```python
from build123d import *

# Parameters (mm, degrees)
SKETCH2_W           = 34
SKETCH2_H           = 34
BOSS_EXTRUDE2_DEPTH = 35
CUT_EXTRUDE6_DEPTH  = 35
SKETCH17_W          = 30
SKETCH17_H          = 30
CUT_EXTRUDE7_DEPTH  = 10
SKETCH18_W          = 30
SKETCH18_H          = 10
CUT_EXTRUDE8_DEPTH  = 30
SKETCH19_R          = 11
CUT_EXTRUDE10_DEPTH = 7
SKETCH20_R          = 11
CUT_EXTRUDE11_DEPTH = 7
SKETCH22_R          = 4
CUT_EXTRUDE12_DEPTH = 30


with BuildPart() as part:
    # Sketch2 → Boss-Extrude2 (new body)
    with BuildSketch(Plane(origin=(0, 0, 0), x_dir=(1, 0, 0), z_dir=(0, 1, 0))):
        Rectangle(SKETCH2_W, SKETCH2_H)
    boss_extrude2 = extrude(amount=BOSS_EXTRUDE2_DEPTH)

    # Sketch16 → Cut-Extrude6 (cut)
    with BuildSketch(Plane.XY.offset(17)):
        Polygon((-17, 35), (-17, 10.991783965), (17, 35), align=None)
    extrude(amount=-CUT_EXTRUDE6_DEPTH, mode=Mode.SUBTRACT)

    # Sketch17 → Cut-Extrude7 (cut)
    with BuildSketch(Plane.XZ):
        Rectangle(SKETCH17_W, SKETCH17_H)
    cut_extrude7 = extrude(amount=-CUT_EXTRUDE7_DEPTH, mode=Mode.SUBTRACT)

    # Mirror6: Boss-Extrude2, Cut-Extrude7 across plane
    add(boss_extrude2.mirror(Plane(origin=(17, 35, -18), x_dir=(0, 0, 1), z_dir=(0.57681494, -0.816874853, 0))))
    add(cut_extrude7.mirror(Plane(origin=(17, 35, -18), x_dir=(0, 0, 1), z_dir=(0.57681494, -0.816874853, 0))), mode=Mode.SUBTRACT)

    # Sketch18 → Cut-Extrude8 (cut)
    with BuildSketch(Plane.ZY.offset(-15)):
        with Locations((0, 5)):
            Rectangle(SKETCH18_W, SKETCH18_H)
    extrude(amount=CUT_EXTRUDE8_DEPTH, mode=Mode.SUBTRACT)

    # Sketch19 → Cut-Extrude10 (cut)
    with BuildSketch(Plane(origin=(0, 0, -17), x_dir=(-1, 0, 0), z_dir=(0, 0, -1))):
        with Locations((0, 22.995891982)):
            Circle(SKETCH19_R)
    extrude(amount=-CUT_EXTRUDE10_DEPTH, mode=Mode.SUBTRACT)

    # Sketch20 → Cut-Extrude11 (cut)
    with BuildSketch(Plane.XY.offset(17)):
        with Locations((0, 22.995891982)):
            Circle(SKETCH20_R)
    extrude(amount=-CUT_EXTRUDE11_DEPTH, mode=Mode.SUBTRACT)

    # Sketch22 → Cut-Extrude12 (cut)
    with BuildSketch(Plane.XY.offset(10)):
        with Locations((0, 22.995891982)):
            Circle(SKETCH22_R)
    extrude(amount=-CUT_EXTRUDE12_DEPTH, mode=Mode.SUBTRACT)


solid = part.part
```
Work out the finished part from the listing and answer in its coordinate system (mm). A direction names the side the tool comes from. Give positions to 0.01 mm unless a question says otherwise; leave off trailing zeros. Write each loop counter-clockwise with the first axis right and the second up, starting at its lowest first coordinate (ties: lowest second). Pieces come first, ordered by that corner, then holes.
(1) The part is cut by section D-D on x = -18. Write down the section's boundary in (y, z), plus the area to 3 significant figures.
Final values:
outline: (11.35, -17) - (41.03, -17) - (41.03, -15) - (13.47, -15) - (13.47, 15) - (41.03, 15) - (41.03, 17) - (11.35, 17) - close
area: 182 mm2
(2) Which of the six approach directions +Z, -Z, +X, -X, +Y, -Y give full straight-line access (tool end or side, diameter ignored) to faces 1 (the flat face through (0, 10, 0)), 2 (the flat face through (0, 18, -10)), 3 (the flat face through (-12.006, 43.176, -0.21)), 4 (the flat face through (17, 17, 0))?
Final values:
face 1: -Y
face 2: -Z
face 3: -X
face 4: +Z, -Z, +X, +Y, -Y
(3) The mould has two halves that part along Z. Classify faces 5 (the flat face through (-8, 15, -17)), 6 (the flat face through (-17, 29, 15)), 7 (the flat face through (0, 5, -15)), 8 (the flat face through (0, 18, 10)): pulls with the +Z half, pulls with the -Z half, needs draft (parallel to the pull), parting line crosses it, or undercut.
Final values:
face 5: pulls with the -Z half
face 6: undercut
face 7: undercut
face 8: pulls with the +Z half
(4) The part is cut by section A-A on y = 9. Write down the section's boundary in (x, z).
Final values:
outline: (-17, -17) - (17, -17) - (17, 17) - (-17, 17) - close; hole (-15, -15) - (15, -15) - (15, 15) - (-15, 15) - close
(5) The part is cut by section C-C on z = -6.5. Write down the section's boundary in (x, y), plus the area to 3 significant figures.
Final values:
outline: (-27.36, 14.67) - (-17, 10.99) - (-17, 0) - (-15, 0) - (-15, 10) - (15, 10) - (15, 0) - (17, 0) - (17, 35) - (-15.98, 46.71) - (-16.65, 44.83) - (-7.23, 41.48) - (-17.27, 13.21) - (-26.69, 16.55) - close; hole circle Ø8 at (0, 23)
area: 913 mm2
(6) Flat-ended cylindrical pins translate along their axes: pin 1 Ø1.5 at (x, z) = (12.5, 1.5) entering from -Y; pin 2 Ø10.5 at (x, y) = (0, 23) entering from +Z; pin 3 Ø1 at (x, z) = (-13.5, -4) entering from +Y. Find the tip coordinate at first contact, or state that the pin passes through.
Final values:
pin 1: stops at y = 10
pin 2: stops at z = 10
pin 3: stops at y = 46.01
(7) The part is cut by section B-B on x = 0. Write down the section's boundary in (y, z), plus the area to 3 significant figures.
Final values:
outline: (0, -17) - (12, -17) - (12, -10) - (19, -10) - (19, 10) - (12, 10) - (12, 17) - (0, 17) - (0, 15) - (10, 15) - (10, -15) - (0, -15) - close; (27, -10) - (34, -10) - (34, -17) - (41.04, -17) - (41.04, 17) - (34, 17) - (34, 10) - (27, 10) - close
area: 627 mm2
(8) Straight lines are drawn through the part: line 1 (Z direction, x = -1.5, y = 2); line 2 (Z direction, x = -7, y = 17); line 3 (Y direction, x = 0.5, z = 9). For each, find the intervals that lie inside material, in ascending order.
Final values:
line 1: z = -17 to -15, 15 to 17
line 2: z = -10 to 10
line 3: y = 10 to 19.03, 26.96 to 40.86
